from build123d import *

# Parameters (mm, degrees)
SKETCH1_R           = 6.35
SKETCH1_R_2         = 2.286
BOSS_EXTRUDE1_DEPTH = 31.75
SKETCH3_R           = 1.27
CUT_EXTRUDE1_DEPTH  = 31.75


with BuildPart() as part:
    # Sketch1 → Boss-Extrude1 (new, symmetric)
    with BuildSketch(Plane.XY):
        Circle(SKETCH1_R)
        Circle(SKETCH1_R_2, mode=Mode.SUBTRACT)
    extrude(amount=BOSS_EXTRUDE1_DEPTH, both=True)

    # Sketch3 → Cut-Extrude1 (cut, symmetric)
    with BuildSketch(Plane(origin=(0, 0, 0), x_dir=(1, 0, 0), z_dir=(0, 1, 0))):
        with Locations(Location((0, 15.875, 0), (0, 0, 270))):
            Circle(SKETCH3_R)
        with Locations(Location((0, -15.875, 0), (0, 0, 270))):
            Circle(SKETCH3_R)
    extrude(amount=CUT_EXTRUDE1_DEPTH, both=True, mode=Mode.SUBTRACT)


solid = part.part
Verification items for the finished model (mm, model axes). Give positions to 0.01 mm unless a question says otherwise; leave off trailing zeros. Loops run counter-clockwise (first coordinate to the right, second up) from the corner with the lowest first, then second, coordinate; pieces in that order, holes last.
1) Depth check by flat-ended pin: pin 1 Ø5 at (y, z) = (4, 17.5) entering from +X; pin 2 Ø3 at (x, z) = (0, 15.875) entering from -Y. Enter the tip coordinate at first touch or a pass-through.
2) Thickness scan on line 1 along Z through (x, y) = (0, -5.35) (3 decimals); line 2 along Y through (x, z) = (0, 0); line 3 along X through (y, z) = (1, -12). Record the ranges inside material, lowest first.
3) Sectioned sample at A-A, the plane x = 0. Enter the section's corners in (y, z) (3 decimals), then the cut area to 3 significant figures.
4) Sectioned sample at C-C, the plane z = -3.5. Enter the section's corners in (x, y), then the cut area to 3 significant figures.
5) Sectioned sample at D-D, the plane y = 4.25. Enter the section's corners in (x, z) (3 decimals).
6) Sectioned sample at B-B, the plane y = 0. Enter the section's corners in (x, z), then the cut area to 3 significant figures.
7) Draft check along Z on faces 1 (the flat face through (3, 0, 31.75)), 2 (the cylindrical face through (-1.38, -6.2, 0.44)), 3 (the cylindrical face through (0.381, -4.096, 17.086)). Enter one of: pulls with the +Z half, pulls with the -Z half, needs draft (parallel to the pull), parting line crosses it, or undercut.
Answers:
1. pin 1: stops at x = 6.17
1. pin 2: stops at y = -6.35
2. line 1: z = -31.75 to -17.145, -14.605 to 14.605, 17.145 to 31.75
2. line 2: y = -6.35 to -2.29, 2.29 to 6.35
2. line 3: x = -6.27 to -2.06, 2.06 to 6.27
3. outline: (-6.35, -31.75) - (-2.286, -31.75) - (-2.286, -17.145) - (-6.35, -17.145) - close; (-6.35, -14.605) - (-2.286, -14.605) - (-2.286, 14.605) - (-6.35, 14.605) - close; (-6.35, 17.145) - (-2.286, 17.145) - (-2.286, 31.75) - (-6.35, 31.75) - close; (2.286, -31.75) - (6.35, -31.75) - (6.35, -17.145) - (2.286, -17.145) - close; (2.286, -14.605) - (6.35, -14.605) - (6.35, 14.605) - (2.286, 14.605) - close; (2.286, 17.145) - (6.35, 17.145) - (6.35, 31.75) - (2.286, 31.75) - close
3. area: 475 mm2
4. outline: circle Ø12.7 at (0, 0); hole circle Ø4.57 at (0, 0)
4. area: 110 mm2
5. outline: (-4.718, -31.75) - (4.718, -31.75) - (4.718, 31.75) - (-4.718, 31.75) - close; hole circle Ø2.54 at (0, -15.875); hole circle Ø2.54 at (0, 15.875)
6. outline: (-6.35, -31.75) - (-2.29, -31.75) - (-2.29, 31.75) - (-6.35, 31.75) - close; (2.29, -31.75) - (6.35, -31.75) - (6.35, 31.75) - (2.29, 31.75) - close
6. area: 516 mm2
7. face 1: pulls with the +Z half
7. face 2: needs draft
7. face 3: undercut
